Geometry check sheet. Reference: drawing and pictorial views, mm from the part's lowest x, y, z. Coordinates: 2 decimals unless noted, no trailing zeros. Loops run counter-clockwise (first coordinate to the right, second up) from the corner with the lowest first, then second, coordinate; pieces in that order, holes last. Notation, with made-up numbers: (-39, -19.75) - (-28, -19.75) arc R28 cw to (-28, 7.25) - close; hole circle Ø6 at (-25.75, -26). An arc over 180 degrees is marked (long way). Write each question's results on one line, items separated by ' | '. Start each with the question number.
1. Cross-section at B-B (x = 38.1). Record the cut outline in (y, z).
2. Cross-section at C-C (x = 103.5). Give the number of separate pieces and of enclosed holes in the cut face.
3. Thickness scan on line 1 (X direction, y = 71, z = 2.75) (1 decimal); line 2 (X direction, y = 21, z = 5.25) (1 decimal); line 3 (Y direction, x = 47, z = 0.5). Record the ranges inside material, lowest first. Write a range as [from, to].
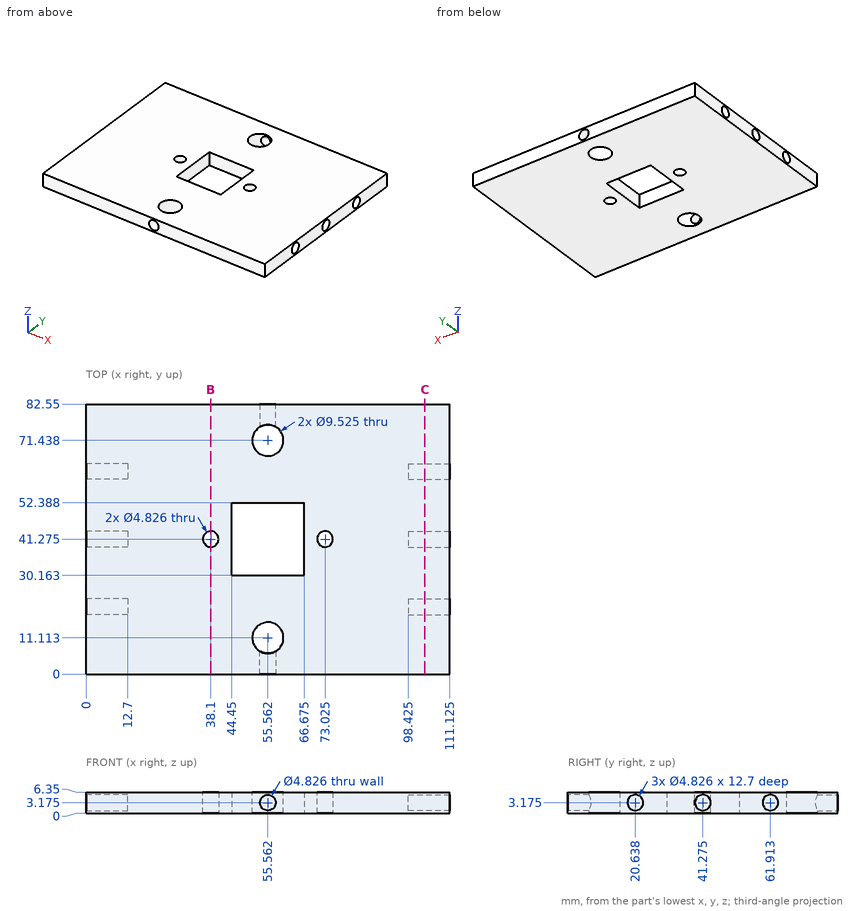
Established:
1) outline: (0, 0) - (38.86, 0) - (38.86, 6.35) - (0, 6.35) - close; (43.69, 0) - (82.55, 0) - (82.55, 6.35) - (43.69, 6.35) - close
2) separate pieces: 1 | enclosed holes: 3
3) line 1: [0, 50.8], [60.3, 111.1] | line 2: [12.7, 98.4] | line 3: [0, 30.16], [52.39, 82.55]
